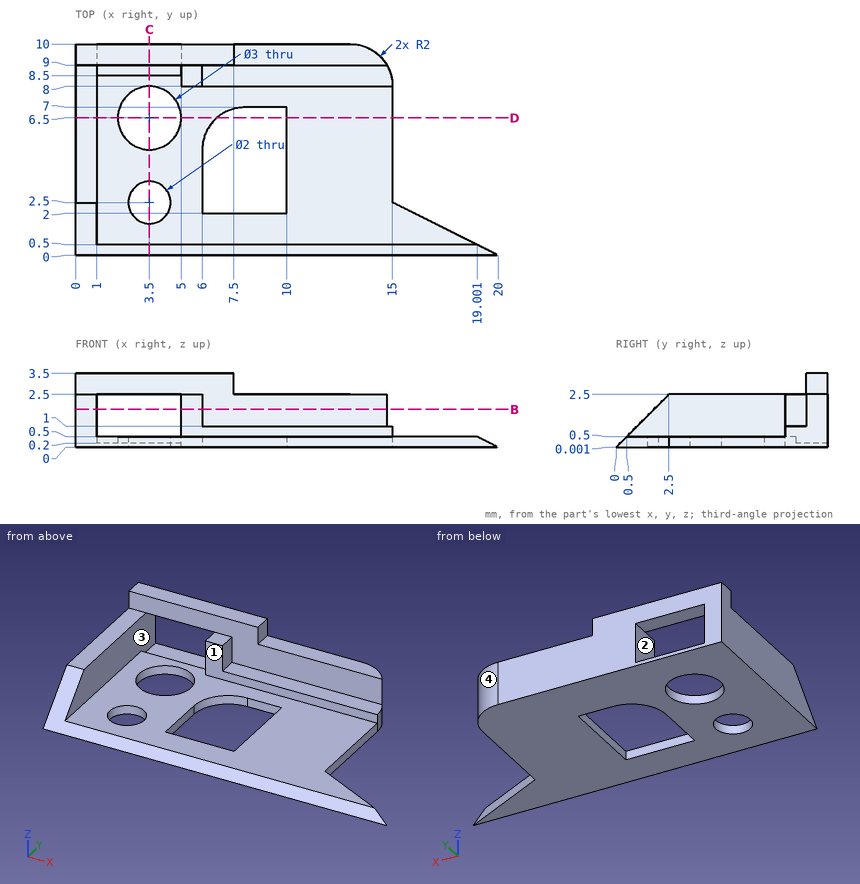
The drawing under review shows one solid part. Ordinate dimensions are in mm from its lowest x, y, z. Coordinates: 2 decimals unless noted, no trailing zeros. Write each loop counter-clockwise with the first axis right and the second up, starting at its lowest first coordinate (ties: lowest second). Pieces come first, ordered by that corner, then holes.
1) To check wall thickness, follow L1, parallel to Y at x = 3.5, z = 0.1; L2, parallel to Y at x = 3.5, z = 0.25; L3, parallel to Z at x = 14, y = 5.5. State the ranges of each line that lie inside material, in increasing order.
2) Add section B-B (z = 1.8). Write out the cut boundary in (x, y).
3) Add section C-C (x = 3.5). State how many separate pieces and enclosed holes the cut face has.
4) Add section D-D (y = 6.5). Write out the cut boundary in (x, z).
5) Insertion check: pin 1 (0.5 mm diameter, centred on y = 8.5, z = 1.5, fed in from +X); pin 2 (1.8 mm diameter, centred on x = 3.5, y = 6.5, fed in from -Z); pin 3 (0.5 mm diameter, centred on x = 5.5, y = 8.5, fed in from +Z); pin 4 (1.2 mm diameter, centred on y = 4, z = 2, fed in from +X). Each pin has a flat end and moves straight along its axis. Give the tip position at first contact, or say it passes through.
6) Mouldability with a two-part tool opening along X and no side actions: class the marked faces 1, 2, 3 and 4 as +X half, -X half, draft (parallel to the pull), parting line (faces both ways), or undercut.
Check result:
1. L1: y = 0.1 to 1.5, 3.5 to 5, 8 to 10
1. L2: y = 0.25 to 1.5, 3.5 to 5, 8 to 8.5
1. L3: z = 0 to 0.5
2. outline: (0, 1.8) - (1, 1.8) - (1, 10) - (0, 10) - close; (5, 8) - (6, 8) - (6, 9) - (14.73, 9) arc R2 ccw to (13, 10) - (5, 10) - close
3. separate pieces: 4
3. enclosed holes: 0
4. outline: (0, 0) - (2, 0) - (2, 0.5) - (1, 0.5) - (1, 2.5) - (0, 2.5) - close; (5, 0) - (6.68, 0) - (6.68, 0.5) - (5, 0.5) - close; (10, 0) - (15, 0) - (15, 0.5) - (10, 0.5) - close
5. pin 1: stops at x = 6
5. pin 2: passes through
5. pin 3: stops at z = 2.5
5. pin 4: stops at x = 1
6. face 1: draft
6. face 2: undercut
6. face 3: undercut
6. face 4: +X half
